Input: part model. Units: mm. Frame: model coordinates. Round coordinates to 2 decimals unless told otherwise and drop trailing zeros. Loops run counter-clockwise (first coordinate to the right, second up) from the corner with the lowest first, then second, coordinate; pieces in that order, holes last. Notation, with made-up numbers: (64.5, 0.25) -> (123.5, 0.25) arc R27 cw to (123.5, 25.25) -> close; hole circle Ø10 at (44, -36). An arc over 180 degrees is marked (long way). Answer as a JSON object with one key per item and string values. Group by question number.
Item 1: Material intervals for line 1 (Y direction, x = 0, z = 0.85); line 2 (X direction, y = 25.4, z = 1) (3 decimals); line 3 (Y direction, x = 1.25, z = 0.8), sorted ascending. Write a range as [from, to].
Item 2: Section query B-B on z = 0.35. Count the separate pieces of the cut face and the enclosed holes in it, and give its area (3 significant figures).
Item 3: Draft query along Y for faces 1 (the cylindrical face through (-0.55, 8.83, 0.78)), 2 (the flat face through (8.061, -2.235, 0.783)), 3 (the flat face through (0, 36, 0)), 4 (the cylindrical face through (2.05, 64.1, 0.78)). Return one class per face: released by +Y, released by -Y, zero draft, split by the parting line, or undercut.
Item 4: Section query C-C on y = 25.4. Return loops of the section in (x, z) (1 decimal), and give its area (3 significant figures).
Item 5: Section query A-A on y = 6.35. Return loops of the section in (x, z) (1 decimal), and give its area (3 significant figures).
Autodesk Inventor part; units mm, degrees
ref_plane "YZ Plane" through (0, 0, 0) normal (1, 0, 0) x (0, 1, 0)
ref_plane "XZ Plane" through (0, 0, 0) normal (0, 1, 0) x (-1, 0, 0)
ref_plane "XY Plane" through (0, 0, 0) normal (0, 0, 1) x (1, 0, 0)
sketch "Sketch1" plane through (0, 0, 0) normal (0, 0, 1) x (1, 0, 0)
  line L0 (0, 0) -> (12.7, 0)
  line L1 (9.525, 0) -> (9.525, 76.2)
  line L2 (9.525, 76.2) -> (-9.525, 76.2)
  line L3 (-9.525, 76.2) -> (-9.525, 0)
  line L4 (-9.525, 0) -> (0, -5.7165)
  line L5 (0, -5.7165) -> (9.525, 0)
  line L6 (-9.525, 0) -> (-5.9562, -4.8471)
  line L7 (-5.9562, -4.8471) -> (0, -5.7165)
  line L8 (0, -5.7165) -> (6.35, -4.8471)
  line L9 (6.35, -4.8471) -> (9.525, 0)
  line L10 (-9.525, 0) -> (0, 0)
  line L11 (0, 0) -> (0, 6.35)
  line L12 (0, 6.35) -> (0, 25.4)
  circle A0 centre (0, 25.4) radius 3.81
  circle A1 centre (0, 6.35) radius 2.54
  line L13 (0, 21.59) -> (0, 8.89)
  line L14 (0, 29.21) -> (0, 67.31)
  circle A2 centre (0, 67.31) radius 3.81
  dimension "d29" = 5.08
  dimension "d7" = 76.2
  dimension "d22" = 6.35
  dimension "d23" = 19.05
  dimension "d28" = 7.62
  dimension "d30" = 38.1
  dimension "d31" = 7.62
extrude "Extrusion5" add sketch "Sketch1" along normal blind 1.5875
fillet "Fillet4" radius 3.175 7 edges at (6.35, -4.8471, 0.7937) (9.525, 0, 0.7937) (0, -5.7165, 0.7937) (-5.9562, -4.8471, 0.7937) (-9.525, 0, 0.7937) (9.525, 76.2, 0.7937) (-9.525, 76.2, 0.7937)
properties part number "PTOPoly"
Solved:
{
 "1": {"line 1": "[-5.68, 3.81], [8.89, 21.59], [29.21, 63.5], [71.12, 76.2]", "line 2": "[-9.525, -3.81], [3.81, 9.525]", "line 3": "[-5.55, 4.14], [8.56, 21.8], [29, 63.71], [70.91, 76.2]"},
 "2": {"separate pieces": "1", "enclosed holes": "3", "area": "1,420 mm²"},
 "3": {"face 1": "undercut", "face 2": "released by -Y", "face 3": "zero draft", "face 4": "undercut"},
 "4": {"outline": "(-9.5, 0) -> (-3.8, 0) -> (-3.8, 1.6) -> (-9.5, 1.6) -> close; (3.8, 0) -> (9.5, 0) -> (9.5, 1.6) -> (3.8, 1.6) -> close", "area": "18.1 mm²"},
 "5": {"outline": "(-9.5, 0) -> (-2.5, 0) -> (-2.5, 1.6) -> (-9.5, 1.6) -> close; (2.5, 0) -> (9.5, 0) -> (9.5, 1.6) -> (2.5, 1.6) -> close", "area": "22.2 mm²"}
}
